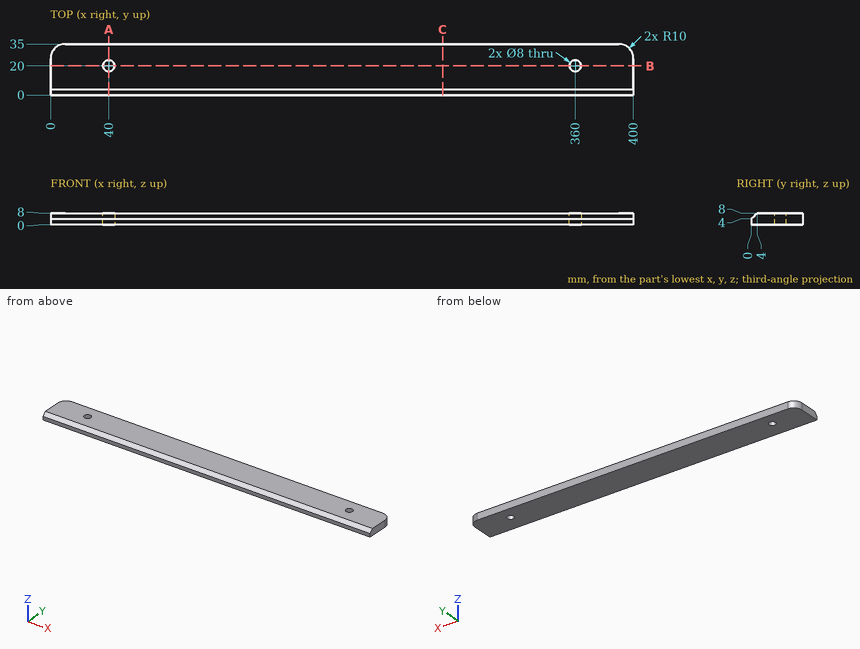
For this review, use the dimensioned drawing (mm, ordinates from the lowest corner) and the shaded views. Coordinates: 2 decimals unless noted, no trailing zeros. Loops run counter-clockwise (first coordinate to the right, second up) from the corner with the lowest first, then second, coordinate; pieces in that order, holes last. Notation, with made-up numbers: (45, 2.25) - (66, 2.25) arc R8 cw to (66, 7.25) - close; hole circle Ø3 at (-4.5, -40). An arc over 180 degrees is marked (long way). Use one line per item in the form item = value. Start each with the question number.
1) To check wall thickness, follow probe 1 along X at (y, z) = (20, 2.5); probe 2 along Y at (x, z) = (360, 2.25); probe 3 along X at (y, z) = (18, 3.75). State the ranges of each line that lie inside material, in increasing order. Write a range as from..to.
2) Take a section at C-C (x = 269). State the section outline as (y, z) points.
3) Take a section at B-B (y = 20). State the section outline as (x, z) points.
4) Take a section at A-A (x = 40). State the section outline as (y, z) points.
5) For pin 1 (6.5 mm diameter, centred on x = 360, y = 20, fed in from +Z), flat-tipped, find the tip position at first contact; note if it passes through.
From the geometry:
q1.probe_1 = 0..36, 44..356, 364..400
q1.probe_2 = 0..16, 24..35
q1.probe_3 = 0..36.54, 43.46..356.54, 363.46..400
q2.outline = (0, 0) - (35, 0) - (35, 8) - (4, 8) - (0, 4) - close
q3.outline = (0, 0) - (36, 0) - (36, 8) - (0, 8) - close; (44, 0) - (356, 0) - (356, 8) - (44, 8) - close; (364, 0) - (400, 0) - (400, 8) - (364, 8) - close
q4.outline = (0, 0) - (16, 0) - (16, 8) - (4, 8) - (0, 4) - close; (24, 0) - (35, 0) - (35, 8) - (24, 8) - close
q5.pin_1 = through
